from build123d import *

# Parameters (mm, degrees)
SHELL3_T           = -2.54
SKETCH2_R          = 15.24
CUT_EXTRUDE2_DEPTH = 63.217039467
SKETCH3_R          = 2.54
CUT_EXTRUDE3_DEPTH = 63.217039467
CIRPATTERN1_COUNT  = 8


with BuildPart() as part:
    # Sketch1 → Revolve1 (revolve)
    with BuildSketch(Plane.XY, mode=Mode.PRIVATE) as revolve1_sk:
        Polygon((0, 0), (0, 50.8), (21.59, 50.8), (21.59, 10.16), (25.4, 10.16), (25.4, 0), align=None)
    revolve(revolve1_sk.sketch.rotate(Axis((0, 0, 0), (0, 1, 0)), 90), axis=Axis((0, 0, 0), (0, 1, 0)))

    # Shell3
    shell3_openings = [part.faces().sort_by_distance(p)[0] for p in [
        (0, 0, 0),
    ]]
    offset(amount=SHELL3_T, openings=shell3_openings, kind=Kind.INTERSECTION)

    # Sketch2 → Cut-Extrude2 (cut, through all)
    with BuildSketch(Plane(origin=(0, 50.8, 0), x_dir=(1, 0, 0), z_dir=(0, 1, 0))):
        with Locations(Location((0, 0, 0), (0, 0, 270))):
            Circle(SKETCH2_R)
    extrude(amount=-CUT_EXTRUDE2_DEPTH, mode=Mode.SUBTRACT)

    # Sketch3 → Cut-Extrude3 (cut, through all)
    with BuildSketch(Plane.XY):
        with Locations(Location((0, 19.05, 0), (0, 0, 90))):
            Circle(SKETCH3_R)
    cut_extrude3 = extrude(amount=-CUT_EXTRUDE3_DEPTH, mode=Mode.SUBTRACT)

    # CirPattern1: Cut-Extrude3 ×8 about axis
    cirpattern1_axis = Axis((0, 50.8, 0), (0, -1, 0))
    for i in range(1, CIRPATTERN1_COUNT):
        add(cut_extrude3.rotate(cirpattern1_axis, i * 360 / CIRPATTERN1_COUNT), mode=Mode.SUBTRACT)


solid = part.part
Here's how the part is built. I have some questions about the finished solid (model axes, mm). A direction names the side the tool comes from. Round coordinates to 2 decimals unless told otherwise and drop trailing zeros. Write each loop counter-clockwise with the first axis right and the second up, starting at its lowest first coordinate (ties: lowest second). Pieces come first, ordered by that corner, then holes. Notation, with made-up numbers: (62, 65.25) -> (86, 65.25) arc R19 ccw to (86, 86.25) -> close; hole circle Ø6 at (15.5, 88.25). An arc over 180 degrees is marked (long way). One line per item, written item: value.
1) Suppose I cut it at B-B on x = 0. List the corners of the cut face in (y, z) for me, plus the area to 3 significant figures.
Filled sheet:
outline: (0, -25.4) -> (10.16, -25.4) -> (10.16, -21.59) -> (16.51, -21.59) -> (16.51, -19.05) -> (7.62, -19.05) -> (7.62, -22.86) -> (0, -22.86) -> close; (0, 22.86) -> (7.62, 22.86) -> (7.62, 19.05) -> (16.51, 19.05) -> (16.51, 21.59) -> (10.16, 21.59) -> (10.16, 25.4) -> (0, 25.4) -> close; (21.59, -21.59) -> (50.8, -21.59) -> (50.8, -15.24) -> (48.26, -15.24) -> (48.26, -19.05) -> (21.59, -19.05) -> close; (21.59, 19.05) -> (48.26, 19.05) -> (48.26, 15.24) -> (50.8, 15.24) -> (50.8, 21.59) -> (21.59, 21.59) -> close
area: 271 mm2
2) If I drill on line 1 (X direction, y = 50, z = 0); line 2 (X direction, y = 2, z = 0); line 3 (Y direction, x = 14.5, z = -5), over which ranges is the centre line in solid material (lowest first)? Write a range as [from, to].
Filled sheet:
line 1: x = [-21.59, -15.24], [15.24, 21.59]
line 2: x = [-25.4, -22.86], [22.86, 25.4]
line 3: y = [48.26, 50.8]
3) I'm going to push flat-ended pins straight in: pin 1 Ø2 at (x, y) = (-16, 32.5) entering from +Z; pin 2 Ø6 at (x, z) = (6.5, -15) entering from -Y; pin 3 Ø8 at (y, z) = (19.05, 0) entering from -X; pin 4 Ø19 at (x, z) = (-1, -2.5) entering from -Y. Where does each tip first touch, or does it pass through?
Filled sheet:
pin 1: stops at z = 15.53
pin 2: stops at y = 7.62
pin 3: stops at x = -21.59
pin 4: passes through
4) Suppose I cut it at D-D on y = 15. List the corners of the cut face in (x, z) for me, plus the area to 3 significant figures.
Filled sheet:
outline: circle Ø43.18 at (0, 0); hole circle Ø38.1 at (0, 0)
area: 324 mm2
5) We'd pull the mould along Y, two halves only. Please class faces 4 (the face through (15.456, 5.009, 20.157)), 5 (the face through (-15, 50.8, 4)), 6 (the face through (-14.375, 16.512, -14.217)): released by +Y, released by -Y, zero draft, split by the parting line, or undercut.
Filled sheet:
face 4: zero draft
face 5: released by +Y
face 6: undercut
6) For faces 1 (the face through (19, 10.16, -11)), 2 (the face through (-13, 48.26, -9)), 3 (the face through (-10, 0, 21)), which set-ups out of +Z, -Z, +X, -X, +Y, -Y let a thin tool reach every point of the face, with its end or its side?
Filled sheet:
face 1: +Y
face 2: -Y
face 3: +Z, -Z, +X, -X, -Y
7) Suppose I cut it at C-C on x = 8.5. List the corners of the cut face in (y, z) for me.
Filled sheet:
outline: (0, -23.94) -> (10.16, -23.94) -> (10.16, -19.85) -> (50.8, -19.85) -> (50.8, -12.65) -> (48.26, -12.65) -> (48.26, -17.05) -> (7.62, -17.05) -> (7.62, -21.22) -> (0, -21.22) -> close; (0, 21.22) -> (7.62, 21.22) -> (7.62, 17.05) -> (48.26, 17.05) -> (48.26, 12.65) -> (50.8, 12.65) -> (50.8, 19.85) -> (10.16, 19.85) -> (10.16, 23.94) -> (0, 23.94) -> close
8) Suppose I cut it at A-A on z = 0. List the corners of the cut face in (x, y) for me.
Filled sheet:
outline: (-25.4, 0) -> (-22.86, 0) -> (-22.86, 7.62) -> (-19.05, 7.62) -> (-19.05, 16.51) -> (-21.59, 16.51) -> (-21.59, 10.16) -> (-25.4, 10.16) -> close; (-21.59, 21.59) -> (-19.05, 21.59) -> (-19.05, 48.26) -> (-15.24, 48.26) -> (-15.24, 50.8) -> (-21.59, 50.8) -> close; (15.24, 48.26) -> (19.05, 48.26) -> (19.05, 21.59) -> (21.59, 21.59) -> (21.59, 50.8) -> (15.24, 50.8) -> close; (19.05, 7.62) -> (22.86, 7.62) -> (22.86, 0) -> (25.4, 0) -> (25.4, 10.16) -> (21.59, 10.16) -> (21.59, 16.51) -> (19.05, 16.51) -> close
